Can you work these out from the drawing? Everything is in mm from the part's minimum corner. A direction names the side the tool comes from. Round coordinates to 2 decimals unless told otherwise and drop trailing zeros. Write each loop counter-clockwise with the first axis right and the second up, starting at its lowest first coordinate (ties: lowest second). Pieces come first, ordered by that corner, then holes. Notation, with made-up numbers: (20.25, -14) - (33.25, -14) arc R25 cw to (33.25, 13) - close; hole circle Ø4 at (-23, 51.25). An arc over 180 degrees is marked (long way). One line per item, written item: value. Start each with the question number.
(1) On a 3-axis mill with a long thin cutter (end or side, diameter ignored), from which of +Z, -Z, +X, -X, +Y, -Y can I reach the whole of each face in a straight line? I mean the marked faces 1 and 2. Say none if no direction works.
(2) I want a section at B-B on y = 13. List the corners of the cut face in (x, z) for me, plus the area to 3 significant figures.
(3) I want a section at A-A on x = 2. List the corners of the cut face in (y, z) for me.
(4) If I drill on L1, parallel to Y at x = 1.5, z = 7; L2, parallel to X at y = 9, z = 8.25; L3, parallel to Z at x = 6.5, y = 6 (1 decimal), over which ranges is the centre line in solid material (lowest first)? Write a range as from..to.
(5) I'm going to push flat-ended pins straight in: pin 1 Ø3 at (x, y) = (8.5, 7) entering from -Z; pin 2 Ø8 at (y, z) = (28, 7) entering from +X. Where does each tip first touch, or does it pass through?
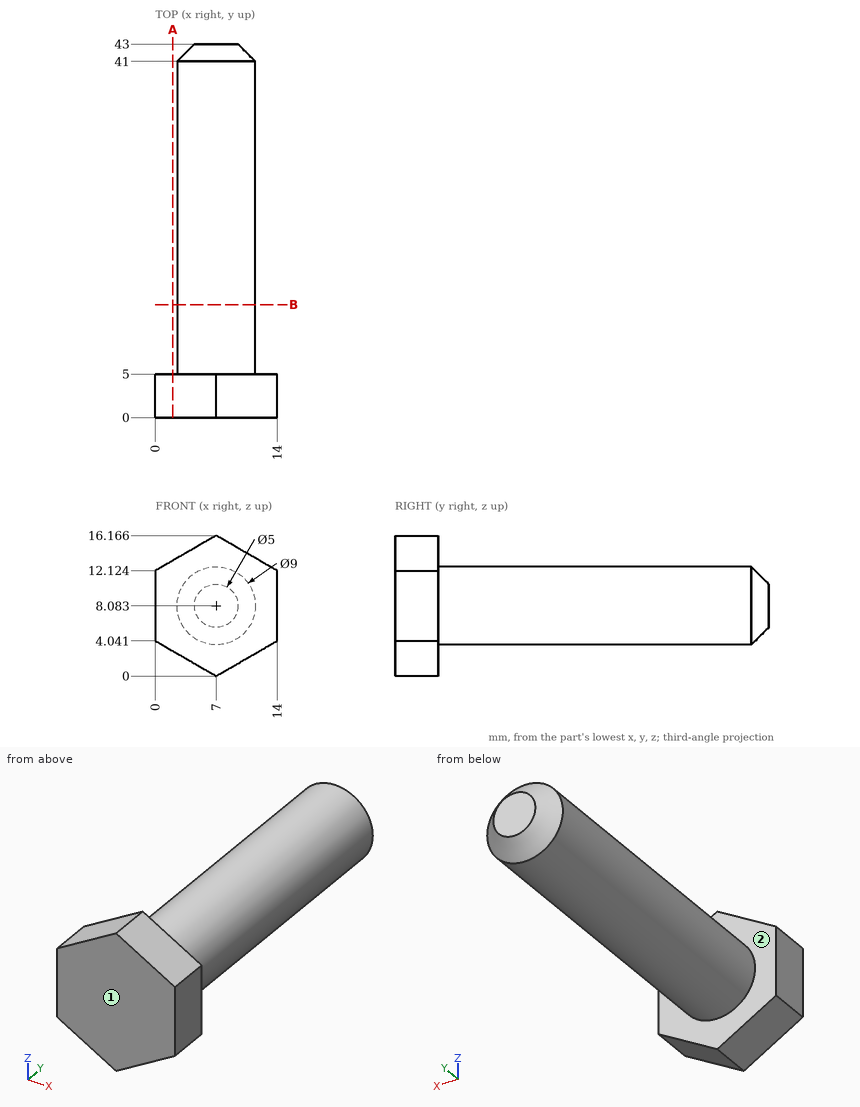
Established:
1. face 1: +Z, -Z, +X, -X, -Y
1. face 2: +Y
2. outline: circle Ø9 at (7, 8.08)
2. area: 63.6 mm2
3. outline: (0, 2.89) - (5, 2.89) - (5, 13.28) - (0, 13.28) - close
4. L1: 0..5
4. L2: 2.5..11.5
4. L3: 3.6..12.6
5. pin 1: z = 3.58
5. pin 2: x = 11.5
